from build123d import *

# Parameters (mm, degrees)
F0_W     = 190.5
F0_H     = 69.85
F1_DEPTH = 10.414


with BuildPart() as f1:
    # F0 (on Top) → F1 (new body)
    with BuildSketch(Plane.XY):
        Polygon((19.05, 0), (0, 0), (0, -19.05), (10.414, -19.05), (10.414, -31.75), (0, -31.75), (0, -44.45), (10.414, -44.45), (10.414, -57.15), (0, -57.15), (0, -69.85), (10.414, -69.85), (10.414, -82.55), (0, -82.55), (0, -95.25), (10.414, -95.25), (10.414, -107.95), (0, -107.95), (0, -120.65), (10.414, -120.65), (10.414, -133.35), (0, -133.35), (0, -146.05), (10.414, -146.05), (10.414, -158.75), (0, -158.75), (0, -177.8), (19.05, -177.8), (19.05, -167.386), (31.75, -167.386), (31.75, -177.8), (44.45, -177.8), (44.45, -167.386), (57.15, -167.386), (57.15, -177.8), (69.85, -177.8), (69.85, -167.386), (82.55, -167.386), (82.55, -177.8), (95.25, -177.8), (95.25, -167.386), (107.95, -167.386), (107.95, -177.8), (120.65, -177.8), (120.65, -167.386), (133.35, -167.386), (133.35, -177.8), (146.05, -177.8), (146.05, -167.386), (158.75, -167.386), (158.75, -177.8), (171.45, -177.8), (171.45, -167.386), (184.15, -167.386), (184.15, -177.8), (196.85, -177.8), (196.85, -167.386), (209.55, -167.386), (209.55, -177.8), (228.6, -177.8), (228.6, -158.75), (218.186, -158.75), (218.186, -146.05), (228.6, -146.05), (228.6, -133.35), (218.186, -133.35), (218.186, -120.65), (228.6, -120.65), (228.6, -107.95), (218.186, -107.95), (218.186, -95.25), (228.6, -95.25), (228.6, -82.55), (218.186, -82.55), (218.186, -69.85), (228.6, -69.85), (228.6, -57.15), (218.186, -57.15), (218.186, -44.45), (228.6, -44.45), (228.6, -31.75), (218.186, -31.75), (218.186, -19.05), (228.6, -19.05), (228.6, 0), (209.55, 0), (209.55, -10.414), (196.85, -10.414), (196.85, 0), (184.15, 0), (184.15, -10.414), (171.45, -10.414), (171.45, 0), (158.75, 0), (158.75, -10.414), (146.05, -10.414), (146.05, 0), (133.35, 0), (133.35, -10.414), (120.65, -10.414), (120.65, 0), (107.95, 0), (107.95, -10.414), (95.25, -10.414), (95.25, 0), (82.55, 0), (82.55, -10.414), (69.85, -10.414), (69.85, 0), (57.15, 0), (57.15, -10.414), (44.45, -10.414), (44.45, 0), (31.75, 0), (31.75, -10.414), (19.05, -10.414), align=None)
        with Locations((114.3, -125.392927)):
            Rectangle(F0_W, F0_H, mode=Mode.SUBTRACT)
        with BuildLine():
            ThreePointArc((66.675, -25.697927), (68.534872, -21.207799), (73.025, -19.347927))
            Line((73.025, -19.347927), (155.575, -19.347927))
            ThreePointArc((155.575, -19.347927), (160.065128, -21.207799), (161.925, -25.697927))
            Line((161.925, -25.697927), (161.925, -28.237927))
            ThreePointArc((161.925, -28.237927), (160.065128, -32.728055), (155.575, -34.587927))
            Line((155.575, -34.587927), (73.025, -34.587927))
            ThreePointArc((73.025, -34.587927), (68.534872, -32.728055), (66.675, -28.237927))
            Line((66.675, -28.237927), (66.675, -25.697927))
        make_face(mode=Mode.SUBTRACT)
    extrude(amount=F1_DEPTH)


solid = f1.part
Verification items for the finished model (mm, model axes). A direction names the side the tool comes from. Round coordinates to 2 decimals unless told otherwise and drop trailing zeros. Loops run counter-clockwise (first coordinate to the right, second up) from the corner with the lowest first, then second, coordinate; pieces in that order, holes last. Notation, with made-up numbers: (-11.5, -18) - (29.5, -18) arc R27 cw to (29.5, 11) - close; hole circle Ø11 at (-18.5, -39.5). An arc over 180 degrees is marked (long way). Use one line per item in the form item = value.
1. Access from +Z, -Z, +X, -X, +Y, -Y to the whole of each face (thin tool, end or side, straight path). Record for faces 4 (the flat face through (51, -167.386, 5)), 5 (the flat face through (223, -158.75, 5)), 6 (the flat face through (10.414, -25, 5)), 7 (the flat face through (133.35, -5, 5)), 8 (the flat face through (113, -160.318, 5)).
A:
face_4 = +Z, -Z, -Y
face_5 = +Z, -Z, +X
face_6 = +Z, -Z, -X
face_7 = +Z, -Z, +Y
face_8 = +Z, -Z
2. Section check D-D on z = 8. Give the number of separate pieces and of enclosed holes in the cut face, and give its area (3 significant figures).
A:
separate_pieces = 1
enclosed_holes = 2
area = 22,200 mm²
3. Gauge pin test, flat ends, axial feed: pin 1 Ø5 at (x, z) = (78, 7.5) entering from +Y; pin 2 Ø2 at (y, z) = (-123, 7) entering from -X. Record the tip position at first contact, or that the pin passes through.
A:
pin_1 = -10.41
pin_2 = 10.41
4. Scan lines: probe 1 along Y at (x, z) = (79, 5.75); probe 2 along Y at (x, z) = (190, 7.75); probe 3 along X at (y, z) = (-122, 7.75). Record each from-to range of solid material in increasing order.
A:
probe_1 = -167.39 to -160.32, -90.47 to -34.59, -19.35 to -10.41
probe_2 = -177.8 to -160.32, -90.47 to 0
probe_3 = 10.41 to 19.05, 209.55 to 218.19
5. Section check A-A on y = -151. Record the cut outline in (x, z), and give its area (3 significant figures).
A:
outline = (10.41, 0) - (19.05, 0) - (19.05, 10.41) - (10.41, 10.41) - close; (209.55, 0) - (218.19, 0) - (218.19, 10.41) - (209.55, 10.41) - close
area = 180 mm²
6. Section check B-B on x = 87. Record the cut outline in (y, z).
A:
outline = (-177.8, 0) - (-160.32, 0) - (-160.32, 10.41) - (-177.8, 10.41) - close; (-90.47, 0) - (-34.59, 0) - (-34.59, 10.41) - (-90.47, 10.41) - close; (-19.35, 0) - (0, 0) - (0, 10.41) - (-19.35, 10.41) - close
7. Section check C-C on x = 194. Record the cut outline in (y, z), and give its area (3 significant figures).
A:
outline = (-177.8, 0) - (-160.32, 0) - (-160.32, 10.41) - (-177.8, 10.41) - close; (-90.47, 0) - (0, 0) - (0, 10.41) - (-90.47, 10.41) - close
area = 1,120 mm²
8. Draft check along X on faces 1 (the flat face through (158.75, -173, 5)), 2 (the flat face through (89, 0, 5)), 3 (the flat face through (0, -38, 5)). Enter one of: pulls with the +X half, pulls with the -X half, needs draft (parallel to the pull), parting line crosses it, or undercut.
A:
face_1 = undercut
face_2 = needs draft
face_3 = pulls with the -X half
